Source: three-view drawing plus pictorial views. Frame: mm from the lowest corner of the part. A direction names the side the tool comes from. Round coordinates to 2 decimals unless told otherwise and drop trailing zeros. Loops run counter-clockwise (first coordinate to the right, second up) from the corner with the lowest first, then second, coordinate; pieces in that order, holes last. Notation, with made-up numbers: M 45.25,8.25 L 83.25,8.25 A19 ccw 83.25,23.25 Z; hole C 85.25,2 d9. An arc over 180 degrees is marked long. Answer as a JSON object with one key per item and string values.
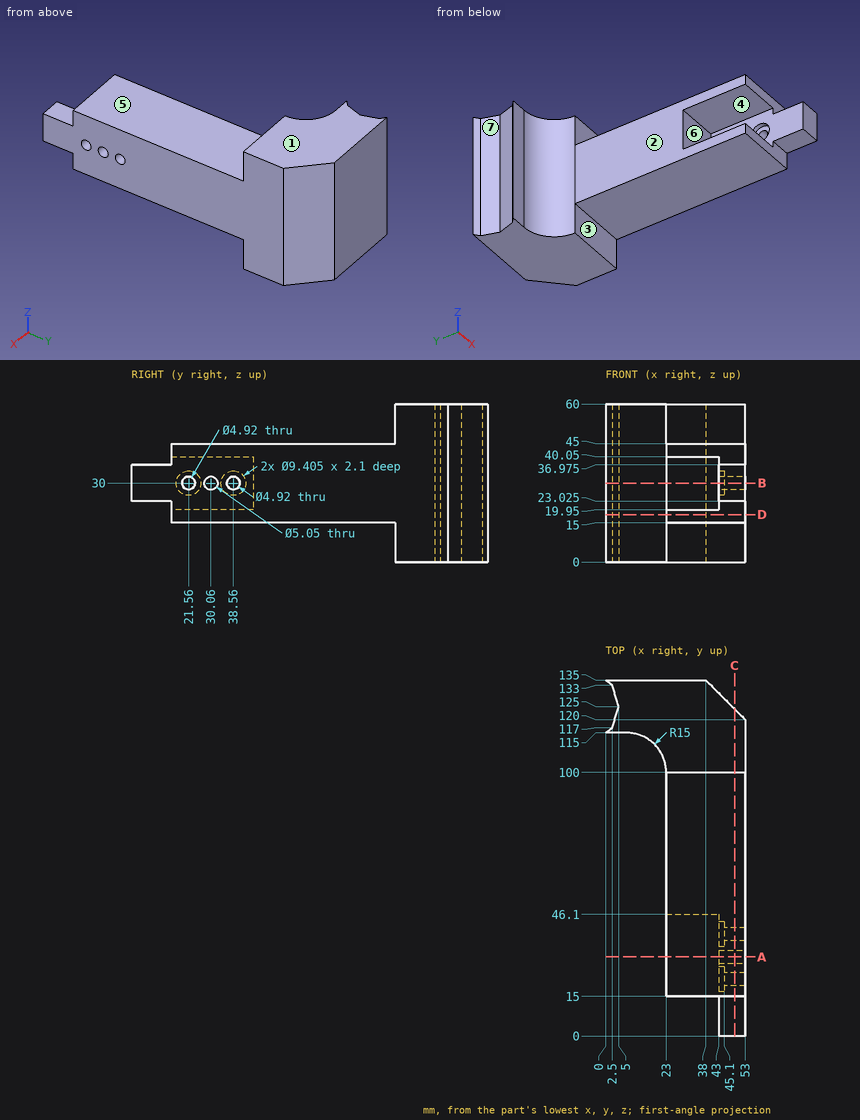
1) Line query: probe 1 along Z at (x, y) = (50.75, 21.56); probe 2 along Z at (x, y) = (30, 24); probe 3 along X at (y, z) = (58, 42). Output: solid intervals per line, ascending.
Geometry results:
{"probe 1": "15 to 27.54, 32.46 to 45", "probe 2": "15 to 19.95, 40.05 to 45", "probe 3": "23 to 53"}
2) Cut plane C-C on x = 49. Return the cut outline in (y, z) (3 decimals), and give its area (3 significant figures).
Geometry results:
{"outline": "M 0,23.025 L 15,23.025 L 15,15 L 100,15 L 100,0 L 124,0 L 124,60 L 100,60 L 100,45 L 15,45 L 15,36.975 L 0,36.975 Z; hole C 21.56,30 d4.92; hole C 30.06,30 d5.05; hole C 38.56,30 d4.92", "area": "4,140 mm2"}
3) Cut plane A-A on y = 30.06. Return the cut outline in (x, z) (3 decimals).
Geometry results:
{"outline": "M 23,15 L 53,15 L 53,27.475 L 43,27.475 L 43,19.95 L 23,19.95 Z; M 23,40.05 L 43,40.05 L 43,32.525 L 53,32.525 L 53,45 L 23,45 Z"}
4) Cut plane D-D on z = 18. Return the cut outline in (x, y).
Geometry results:
{"outline": "M 0,115 L 8,115 A15 cw 23,100 L 23,15 L 53,15 L 53,120 L 38,135 L 0,135 L 2.5,133 L 5,125 L 2.5,117 Z"}
5) Cut plane B-B on z = 30. Count the separate pieces of the cut face and the enclosed holes in it, and give its area (3 significant figures).
Geometry results:
{"separate pieces": "4", "enclosed holes": "0", "area": "3,290 mm2"}
6) Pull-direction query (Z, two-part tool) for the marked faces 5, 6 and 7; classes: +Z half, -Z half, draft (parallel to the pull), parting line (faces both ways), or undercut.
Geometry results:
{"face 5": "+Z half", "face 6": "undercut", "face 7": "draft"}
7) First-contact query: pin 1 (4.5 mm diameter, centred on x = 38, z = 10.5, fed in from -Y); pin 2 (15 mm diameter, centred on x = 37, y = 64.5, fed in from -Z); pin 3 (3 mm diameter, centred on x = 47.5, y = 4, fed in from +Z) (3 decimals); pin 4 (5 mm diameter, centred on x = 15, y = 107.5, fed in from -Z). Flat tips, straight axial feed; report the tip coordinate or a pass-through.
Geometry results:
{"pin 1": "y = 100", "pin 2": "z = 15", "pin 3": "z = 36.975", "pin 4": "through"}
8) Set-up query: the marked faces 1, 2, 3 and 4. Return all of +Z, -Z, +X, -X, +Y, -Y with unobstructed straight access to the full face (end or side cutting, diameter ignored); none if empty.
Geometry results:
{"face 1": "+Z, +X, -X, +Y, -Y", "face 2": "+Z, -Z, -X, -Y", "face 3": "-Z, +X, -X, -Y", "face 4": "-X, -Y"}
